```python
from build123d import *

# Parameters (mm, degrees)
SKETCH1_W           = 130
SKETCH1_H           = 80
BOSS_EXTRUDE1_DEPTH = 1.5
FILLET1_R           = 4
SKETCH4_W           = 98
SKETCH4_H           = 57
CUT_EXTRUDE1_DEPTH  = 6
SKETCH6_W           = 7
SKETCH6_H           = 64
CUT_EXTRUDE3_DEPTH  = 10
FILLET3_R           = 4
CHAMFER1_SIZE       = 1


with BuildPart() as part:
    # Sketch1 → Boss-Extrude1 (new body)
    with BuildSketch(Plane.XY):
        Rectangle(SKETCH1_W, SKETCH1_H)
    extrude(amount=BOSS_EXTRUDE1_DEPTH)

    # Fillet1
    fillet1_edges = [part.edges().sort_by_distance(p)[0] for p in [
        (65, -40, 0.75),
        (-65, -40, 0.75),
        (-65, 40, 0.75),
        (65, 40, 0.75),
    ]]
    fillet(fillet1_edges, radius=FILLET1_R)

    # Sketch3 → CSK for M3 Flat Countersunk Head Screw1 (revolve, cut)
    with BuildSketch(Plane(origin=(-61, 36, 1.5), x_dir=(0, -1, 0), z_dir=(1, 0, 0))):
        Polygon((0, 0), (0, 1.5), (1.8, 1.5), (1.8, 1.35), (3.15, 0), align=None)
    csk_for_m3_flat_countersunk_head_screw1 = revolve(axis=Axis((-61, 36, 7.85), (0, 0, -1)), mode=Mode.SUBTRACT)

    # Mirror1: CSK for M3 Flat Countersunk Head Screw1 across plane
    add(csk_for_m3_flat_countersunk_head_screw1.mirror(Plane(origin=(0, 0, 0), x_dir=(0, 0, 1), z_dir=(1, 0, 0))), mode=Mode.SUBTRACT)

    # Mirror2: CSK for M3 Flat Countersunk Head Screw1 across plane
    add(csk_for_m3_flat_countersunk_head_screw1.mirror(Plane.ZX), mode=Mode.SUBTRACT)

    # Mirror2 copy 1 sketch → Mirror2 copy 1 (revolve, cut)
    with BuildSketch(Plane(origin=(61, -36, 1.5), x_dir=(0, 1, 0), z_dir=(-1, 0, 0))):
        Polygon((0, 0), (0, 1.5), (1.8, 1.5), (1.8, 1.35), (3.15, 0), align=None)
    revolve(axis=Axis((61, -36, 7.85), (0, 0, -1)), mode=Mode.SUBTRACT)

    # Sketch4 → Cut-Extrude1 (cut)
    with BuildSketch(Plane.XY.offset(1.5)):
        with Locations((0, 2.45)):
            Rectangle(SKETCH4_W, SKETCH4_H)
    extrude(amount=-CUT_EXTRUDE1_DEPTH, mode=Mode.SUBTRACT)

    # Sketch6 → Cut-Extrude3 (cut)
    with BuildSketch(Plane.XY.offset(1.5)):
        with Locations((61.5, 0)):
            Rectangle(SKETCH6_W, SKETCH6_H)
    cut_extrude3 = extrude(amount=-CUT_EXTRUDE3_DEPTH, mode=Mode.SUBTRACT)

    # Mirror6: Cut-Extrude3 across plane
    add(cut_extrude3.mirror(Plane(origin=(0, 0, 0), x_dir=(0, 0, 1), z_dir=(1, 0, 0))), mode=Mode.SUBTRACT)

    # Fillet3
    fillet3_edges = [part.edges().sort_by_distance(p)[0] for p in [
        (65, -32, 0.75),
        (65, 32, 0.75),
        (-65, -32, 0.75),
        (-65, 32, 0.75),
    ]]
    fillet(fillet3_edges, radius=FILLET3_R - 0.0001)  # a hair under: the kernel refuses the full size

    # Chamfer1
    chamfer1_edges = [part.edges().sort_by_distance(p)[0] for p in [
        (-49, 2.45, 1.5),
        (0, -26.05, 1.5),
        (49, 2.45, 1.5),
        (0, 30.95, 1.5),
    ]]
    chamfer(chamfer1_edges, length=CHAMFER1_SIZE)


solid = part.part
```
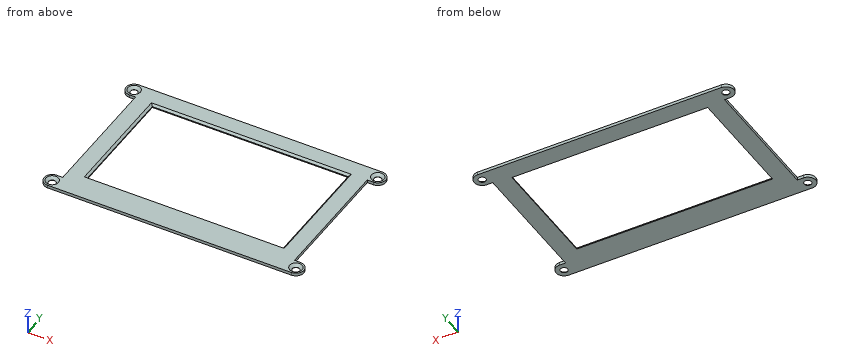
Work out the finished part from the listing and answer in its coordinate system (mm). Round coordinates to 2 decimals unless told otherwise and drop trailing zeros. Loops run counter-clockwise (first coordinate to the right, second up) from the corner with the lowest first, then second, coordinate; pieces in that order, holes last.
(1) Find the intervals of material crossed by L1, parallel to Y at x = -61, z = 0.1; L2, parallel to X at y = -36, z = 0.1; L3, parallel to Y at x = -36, z = 0.3, in increasing order.
Computed values:
L1: y = -40 to -37.8, -34.2 to -32, 32 to 34.2, 37.8 to 40
L2: x = -65 to -62.8, -59.2 to 59.2, 62.8 to 65
L3: y = -40 to -26.05, 30.95 to 40
(2) Each of these flat-tipped pins is pushed along its axis until it touches: P1, Ø4, axis at x = 61, y = -36, coming from the +Z side; P2, Ø4.5, axis at x = -61, y = -36, coming from the +Z side; P3, Ø0.6, axis at y = -9, z = 0.5, coming from the +X side. Where does it stop, or does it pass through?
Computed values:
P1: stops at z = 0.35
P2: stops at z = 0.6
P3: stops at x = 58
(3) The part is cut by section B-B, the plane x = 6.5. Give the vertices of the cut face in (y, z), and give its area (3 significant figures).
Computed values:
outline: (-40, 0) - (-26.05, 0) - (-26.05, 0.5) - (-27.05, 1.5) - (-40, 1.5) - close; (30.95, 0) - (40, 0) - (40, 1.5) - (31.95, 1.5) - (30.95, 0.5) - close
area: 33.5 mm2
(4) The part is cut by section A-A, the plane y = 25. Give the vertices of the cut face in (x, z), and give its area (3 significant figures).
Computed values:
outline: (-58, 0) - (-49, 0) - (-49, 0.5) - (-50, 1.5) - (-58, 1.5) - close; (49, 0) - (58, 0) - (58, 1.5) - (50, 1.5) - (49, 0.5) - close
area: 26.0 mm2
(5) The part is cut by section C-C, the plane z = 0.95. Give the number of separate pieces and of enclosed holes in the cut face, and give its area (3 significant figures).
Computed values:
separate pieces: 1
enclosed holes: 5
area: 3,670 mm2
